from build123d import *

# Parameters (mm, degrees)
SKETCH_1_R          = 3.05
SKETCH_1_R_2        = 2
EXTRUDE_1_DEPTH     = 2
SKETCH_2_R          = 1
CUT_EXTRUDE_1_DEPTH = 61.911082735
CHAMFER_1_SIZE      = 4
CUT_EXTRUDE_2_DEPTH = 61.911082735
FILLET_1_R          = 1
FILLET_2_R          = 2


with BuildPart() as part:
    # 草图1 → 凸台-拉伸1 (new, symmetric)
    with BuildSketch(Plane.XY):
        Polygon((-39, 10), (39, 10), (39, 14.6), (59, 14.6), (59, -5.4), (39, -5.4), (39, -10), (-39, -10), (-39, -5.4), (-59, -5.4), (-59, 14.6), (-39, 14.6), align=None)
        with Locations((-29, 0)):
            Circle(SKETCH_1_R, mode=Mode.SUBTRACT)
        with Locations((29, 0)):
            Circle(SKETCH_1_R, mode=Mode.SUBTRACT)
        with Locations((-49, 4.6)):
            Circle(SKETCH_1_R_2, mode=Mode.SUBTRACT)
        with Locations(Location((49, 4.6, 0), (0, 0, 180))):
            Circle(SKETCH_1_R_2, mode=Mode.SUBTRACT)
    extrude(amount=EXTRUDE_1_DEPTH, both=True)

    # 草图2 → 切除-拉伸1 (cut, through all)
    with BuildSketch(Plane.XY.offset(2)):
        with Locations((-38, 10)):
            Circle(SKETCH_2_R)
        with Locations((-40, -5.4)):
            Circle(SKETCH_2_R)
        with Locations((38, 10)):
            Circle(SKETCH_2_R)
        with Locations((40, -5.4)):
            Circle(SKETCH_2_R)
        Polygon((-24.857864376, 10), (-19.857864376, 5), (19.857864376, 5), (24.857864376, 10), align=None)
    extrude(amount=-CUT_EXTRUDE_1_DEPTH, mode=Mode.SUBTRACT)

    # 倒角1
    chamfer_1_edges = [part.edges().sort_by_distance(p)[0] for p in [
        (39, 14.6, 0),
        (59, 14.6, 0),
        (59, -5.4, 0),
        (39, -10, 0),
        (-39, -10, 0),
        (-59, -5.4, 0),
        (-59, 14.6, 0),
        (-39, 14.6, 0),
    ]]
    chamfer(chamfer_1_edges, length=CHAMFER_1_SIZE)

    # 草图3 → 切除-拉伸2 (cut, through all)
    with BuildSketch(Plane.XY.offset(2)):
        Polygon((-14.857864376, 0), (-20.357864376, -5.5), (20.357864376, -5.5), (14.857864376, 0), align=None)
    extrude(amount=-CUT_EXTRUDE_2_DEPTH, mode=Mode.SUBTRACT)

    # 圆角1
    fillet_1_edges = [part.edges().sort_by_distance(p)[0] for p in [
        (20.357864376, -5.5, 0),
        (-20.357864376, -5.5, 0),
    ]]
    fillet(fillet_1_edges, radius=FILLET_1_R)

    # 圆角2
    fillet_2_edges = [part.edges().sort_by_distance(p)[0] for p in [
        (-14.857864376, 0, 0),
        (14.857864376, 0, 0),
        (19.857864376, 5, 0),
        (-19.857864376, 5, 0),
    ]]
    fillet(fillet_2_edges, radius=FILLET_2_R)


solid = part.part
Part model, mm, in its own coordinate system. A direction names the side the tool comes from. Coordinates: 2 decimals unless noted, no trailing zeros. Loops run counter-clockwise (first coordinate to the right, second up) from the corner with the lowest first, then second, coordinate; pieces in that order, holes last. Notation, with made-up numbers: M 28.5,24.25 L 37.5,24.25 A14 ccw 37.5,42.25 Z; hole C 89.5,27.5 d6. An arc over 180 degrees is marked long. Use a Markdown table: item, result. Add a question column.
Q1. Cut at B-B (x = -49). Write the cut outline in (y, z).
Q2. Cut at A-A (x = 29). Write the cut outline in (y, z), and give its area (3 significant figures).
Q3. Cut at C-C (z = 1). Give the number of separate pieces and of enclosed holes in the cut face, and give its area (3 significant figures).
Q4. Mould opens along Y. For faces 4 (the flat face through (-37, -8, 0)), 5 (the cylindrical face through (-47.153, 3.834, -0.028)), 6 (the flat face through (0, -5.5, 0)), 7 (the flat face through (-59, 5, 0)) say: +Y half, -Y half, draft (parallel to the pull), parting line (faces both ways), or undercut.
Q5. Probe L1, parallel to Y at x = -29, z = -0.9; L2, parallel to X at y = 1, z = -0.1; L3, parallel to Y at x = -4, z = -0.8. List the from-to ranges inside material, lowest first.
Q6. Pin check, flat tips, straight feed: P1, Ø0.5, axis at y = -5.5, z = -0.5, coming from the +X side; P2, Ø2, axis at x = -49, z = 0.5, coming from the -Y side; P3, Ø1.5, axis at x = 3, z = 0, coming from the +Y side. Stop position of each tip, or through.
Q7. Which spindle directions (+Z, -Z, +X, -X, +Y, -Y) get a long thin tool onto all of the face, cutting with end or side? Do faces 1 (the flat face through (-22.68, 7.82, 0.03)), 2 (the flat face through (17.07, -2.21, 0.03)), 3 (the flat face through (57, -3.4, 0)). Say none if no direction does.
Worked out:
| question | item | result |
|---|---|---|
| 1 | outline | M -5.4,-2 L 2.6,-2 L 2.6,2 L -5.4,2 Z; M 6.6,-2 L 14.6,-2 L 14.6,2 L 6.6,2 Z |
| 2 | outline | M -10,-2 L -3.05,-2 L -3.05,2 L -10,2 Z; M 3.05,-2 L 10,-2 L 10,2 L 3.05,2 Z |
| 2 | area | 55.6 mm2 |
| 3 | separate pieces | 1 |
| 3 | enclosed holes | 5 |
| 3 | area | 1,790 mm2 |
| 4 | face 4 | -Y half |
| 4 | face 5 | undercut |
| 4 | face 6 | undercut |
| 4 | face 7 | draft |
| 5 | L1 | y = -10 to -3.05, 3.05 to 10 |
| 5 | L2 | x = -59 to -31.88, -26.12 to 26.12, 31.88 to 59 |
| 5 | L3 | y = -10 to -5.5, 0 to 5 |
| 6 | P1 | stops at x = 55.15 |
| 6 | P2 | stops at y = -5.4 |
| 6 | P3 | stops at y = 5 |
| 7 | face 1 | +Z, -Z, +Y |
| 7 | face 2 | +Z, -Z |
| 7 | face 3 | +Z, -Z, +X, -Y |
